from build123d import *

# Parameters (mm, degrees)
SKETCH1_R           = 17.78
SKETCH1_R_2         = 2.5527
SKETCH1_R_3         = 9.525
BOSS_EXTRUDE1_DEPTH = 15.9766


with BuildPart() as part:
    # Sketch1 → Boss-Extrude1 (new body)
    with BuildSketch(Plane(origin=(0, 0, 0), x_dir=(1, 0, 0), z_dir=(0, 1, 0))):
        Circle(SKETCH1_R)
        with Locations((0, 13.97)):
            Circle(SKETCH1_R_2, mode=Mode.SUBTRACT)
        with Locations((9.878281733, 9.878281733)):
            Circle(SKETCH1_R_2, mode=Mode.SUBTRACT)
        with Locations((13.97, 0)):
            Circle(SKETCH1_R_2, mode=Mode.SUBTRACT)
        with Locations((9.878281733, -9.878281733)):
            Circle(SKETCH1_R_2, mode=Mode.SUBTRACT)
        with Locations((0, -13.97)):
            Circle(SKETCH1_R_2, mode=Mode.SUBTRACT)
        with Locations((-9.878281733, -9.878281733)):
            Circle(SKETCH1_R_2, mode=Mode.SUBTRACT)
        with Locations((-13.97, 0)):
            Circle(SKETCH1_R_2, mode=Mode.SUBTRACT)
        with Locations((-9.878281733, 9.878281733)):
            Circle(SKETCH1_R_2, mode=Mode.SUBTRACT)
        Circle(SKETCH1_R_3, mode=Mode.SUBTRACT)
    extrude(amount=BOSS_EXTRUDE1_DEPTH)


solid = part.part
Can you work these out from the model? Positions are in its coordinate system, mm. Round coordinates to 2 decimals unless told otherwise and drop trailing zeros. Loops run counter-clockwise (first coordinate to the right, second up) from the corner with the lowest first, then second, coordinate; pieces in that order, holes last. Notation, with made-up numbers: (85.25, 23) - (107.25, 23) arc R10 cw to (107.25, 28) - close; hole circle Ø1 at (-32, 13.5). An arc over 180 degrees is marked (long way). Write item = value, one per line. Start each with the question number.
(1) If we section it at D-D (z = 13.97): Please give me the cut outline in (x, y).
(2) If we mould it in two halves opening along Z, with no side actions, what happens to faces 1 (the face through (7.7, 15.977, 7.7)), 2 (the face through (11.06, 7.88, 12.14)), 3 (the face through (-3.85, 7.88, 17.36))? For each: released by +Z, released by -Z, zero draft, split by the parting line, or undercut.
(3) If we section it at B-B (x = 0): Please give me the cut outline in (y, z) (3 decimals).
(4) If I drill on probe 1 along X at (y, z) = (10.75, 0) (3 decimals); probe 2 along Z at (x, y) = (-1, 5.75), over which ranges is the centre line in solid material (lowest first)? Write a range as [from, to].
(5) For P1, Ø3, axis at y = 2.5, z = 11, coming from the +X side; P2, Ø3, axis at x = 6, y = 3.5, coming from the -Z side; P3, Ø1, axis at x = 6.5, y = 5.5, coming from the -Z side, each with a flat end and sliding along its axis, tell me the tip position at first contact or that it passes through.
(6) If we section it at C-C (x = 4): Please give me the cut outline in (y, z).
(7) If we section it at A-A (z = 0): Please give me the cut outline in (x, y) (3 decimals), and give its area (3 significant figures).
Ans:
q1.outline = (-11, 0) - (-2.55, 0) - (-2.55, 15.98) - (-11, 15.98) - close; (2.55, 0) - (11, 0) - (11, 15.98) - (2.55, 15.98) - close
q2.face_1 = zero draft
q2.face_2 = undercut
q2.face_3 = split by the parting line
q3.outline = (0, -17.78) - (15.977, -17.78) - (15.977, -16.523) - (0, -16.523) - close; (0, -11.417) - (15.977, -11.417) - (15.977, -9.525) - (0, -9.525) - close; (0, 9.525) - (15.977, 9.525) - (15.977, 11.417) - (0, 11.417) - close; (0, 16.523) - (15.977, 16.523) - (15.977, 17.78) - (0, 17.78) - close
q4.probe_1 = [-17.78, -16.523], [-11.417, -9.525], [9.525, 11.417], [16.523, 17.78]
q4.probe_2 = [-17.75, -16.32], [-11.62, -9.47], [9.47, 11.62], [16.32, 17.75]
q5.P1 = 15.03
q5.P2 = -17.2
q5.P3 = -16.74
q6.outline = (0, -17.32) - (15.98, -17.32) - (15.98, -8.64) - (0, -8.64) - close; (0, 8.64) - (15.98, 8.64) - (15.98, 17.32) - (0, 17.32) - close
q7.outline = (-17.78, 0) - (-16.523, 0) - (-16.523, 15.977) - (-17.78, 15.977) - close; (-11.417, 0) - (-9.525, 0) - (-9.525, 15.977) - (-11.417, 15.977) - close; (9.525, 0) - (11.417, 0) - (11.417, 15.977) - (9.525, 15.977) - close; (16.523, 0) - (17.78, 0) - (17.78, 15.977) - (16.523, 15.977) - close
q7.area = 101 mm²
